For this review, take the finished solid that the model builds, in its own axes (mm). A direction names the side the tool comes from. Coordinates: 2 decimals unless noted, no trailing zeros. Loops run counter-clockwise (first coordinate to the right, second up) from the corner with the lowest first, then second, coordinate; pieces in that order, holes last. Notation, with made-up numbers: (-10, 80.5) -> (32, 80.5) arc R21 cw to (32, 85.5) -> close; hole circle Ø8 at (-3, 81). An arc over 180 degrees is marked (long way). Answer in a Markdown table with one row per item.
from build123d import *

# Parameters (mm, degrees)
SKETCH_1_W           = 27.3
SKETCH_1_H           = 27.8
EXTRUDE_1_DEPTH      = 1.6
SKETCH_2_R           = 0.6
EXTRUDE_2_DEPTH      = 4.9
EXTRUDE_2_DEPTH_BACK = 2
SKETCH_3_W           = 27.3
SKETCH_3_H           = 19.2
EXTRUDE_3_DEPTH      = 1.6
SKETCH_4_W           = 14
SKETCH_4_H           = 4
EXTRUDE_4_DEPTH      = 1.4


with BuildPart() as part:
    # 草图1 → 凸台-拉伸1 (new body)
    with BuildSketch(Plane(origin=(0, 0, 0), x_dir=(1, 0, 0), z_dir=(0, 1, 0))):
        with Locations((13.65, 13.9)):
            Rectangle(SKETCH_1_W, SKETCH_1_H)
    extrude(amount=EXTRUDE_1_DEPTH)

    # 草图2 → 凸台-拉伸2 (add, two sides)
    with BuildSketch(Plane.XZ) as extrude_2_sk:
        with Locations((14.92, -26.3)):
            Circle(SKETCH_2_R)
        with Locations((12.38, -26.3)):
            Circle(SKETCH_2_R)
    extrude(amount=EXTRUDE_2_DEPTH)
    extrude(extrude_2_sk.sketch, amount=-EXTRUDE_2_DEPTH_BACK)

    # 草图3 → 凸台-拉伸3 (add)
    with BuildSketch(Plane(origin=(0, 1.6, 0), x_dir=(1, 0, 0), z_dir=(0, 1, 0))):
        with Locations((13.65, 13.6)):
            Rectangle(SKETCH_3_W, SKETCH_3_H)
    extrude(amount=EXTRUDE_3_DEPTH)

    # 草图4 → 凸台-拉伸4 (add)
    with BuildSketch(Plane(origin=(0, 1.6, 0), x_dir=(1, 0, 0), z_dir=(0, 1, 0))):
        with Locations((13.65, 2)):
            Rectangle(SKETCH_4_W, SKETCH_4_H)
    extrude(amount=EXTRUDE_4_DEPTH)


solid = part.part
Item 1: Take a section at D-D, the plane x = 14.92. State the section outline as (y, z) points.
Worked answers:
| item | result |
|---|---|
| outline | (-4.9, -26.9) -> (0, -26.9) -> (0, -27.8) -> (1.6, -27.8) -> (1.6, -26.9) -> (2, -26.9) -> (2, -25.7) -> (1.6, -25.7) -> (1.6, -23.2) -> (3.2, -23.2) -> (3.2, -4) -> (3, -4) -> (3, 0) -> (0, 0) -> (0, -25.7) -> (-4.9, -25.7) -> close |
Item 2: Take a section at A-A, the plane x = 25.5. State the section outline as (y, z) points.
Worked answers:
| item | result |
|---|---|
| outline | (0, -27.8) -> (1.6, -27.8) -> (1.6, -23.2) -> (3.2, -23.2) -> (3.2, -4) -> (1.6, -4) -> (1.6, 0) -> (0, 0) -> close |
Item 3: Insertion check: pin 1 (2 mm diameter, centred on x = 14.5, z = -1, fed in from +Y); pin 2 (1.3 mm diameter, centred on x = 12.5, z = -26.5, fed in from +Y); pin 3 (2 mm diameter, centred on x = 23.5, z = -2, fed in from +Y); pin 4 (1.3 mm diameter, centred on x = 20, y = 2, fed in from +Z). Each pin has a flat end and moves straight along its axis. Give the tip position at first contact, or say it passes through.
Worked answers:
| item | result |
|---|---|
| pin 1 | y = 3 |
| pin 2 | y = 2 |
| pin 3 | y = 1.6 |
| pin 4 | z = 0 |
Item 4: Take a section at C-C, the plane y = -2.5. State the section outline as (x, z) points, and give its area (3 significant figures).
Worked answers:
| item | result |
|---|---|
| outline | circle Ø1.2 at (12.38, -26.3); circle Ø1.2 at (14.92, -26.3) |
| area | 2.26 mm² |
Item 5: The part is to be moulded in two halves that separate along X. For faces 5 (the cylindrical face through (14.79, 1.797, -26.886)), 6 (the flat face through (12.4, 2, -26.3)), 7 (the flat face through (6.65, 2, -2)), say which applies: +X half, -X half, draft (parallel to the pull), parting line (faces both ways), or undercut.
Worked answers:
| item | result |
|---|---|
| face 5 | undercut |
| face 6 | draft |
| face 7 | -X half |
Item 6: Take a section at B-B, the plane z = -26.3. State the section outline as (x, y) points.
Worked answers:
| item | result |
|---|---|
| outline | (0, 0) -> (11.78, 0) -> (11.78, -4.9) -> (12.98, -4.9) -> (12.98, 0) -> (14.32, 0) -> (14.32, -4.9) -> (15.52, -4.9) -> (15.52, 0) -> (27.3, 0) -> (27.3, 1.6) -> (15.52, 1.6) -> (15.52, 2) -> (14.32, 2) -> (14.32, 1.6) -> (12.98, 1.6) -> (12.98, 2) -> (11.78, 2) -> (11.78, 1.6) -> (0, 1.6) -> close |
Item 7: For L1, parallel to Y at x = 18.75, z = -13.5; L2, parallel to Y at x = 22.5, z = -24.5; L3, parallel to X at y = -0.25, z = -26, list the stretches that pass through material, from the lowest coordinate up.
Worked answers:
| item | result |
|---|---|
| L1 | 0 to 3.2 |
| L2 | 0 to 1.6 |
| L3 | 11.86 to 12.9, 14.4 to 15.44 |
Item 8: For faces 1 (the flat face through (15, 2, -26)), 2 (the flat face through (14, 3, -2)), 3 (the cylindrical face through (12.25, -2.416, -26.886)), 4 (the cylindrical face through (12.25, 1.797, -26.886)), list the 3-axis set-ups (+Z, -Z, +X, -X, +Y, -Y) from which the entire face can be reached by the end or side of a thin tool; tool diameter is ignored.
Worked answers:
| item | result |
|---|---|
| face 1 | -Z, +X, -X, +Y |
| face 2 | +Z, +X, -X, +Y |
| face 3 | -Y |
| face 4 | +Y |
